The drawing under review shows one solid part. Ordinate dimensions are in mm from its lowest x, y, z. A direction names the side the tool comes from. Round coordinates to 2 decimals unless told otherwise and drop trailing zeros. Order: outer loops, then holes, each group sorted by start corner. A loop starts at its lowest first (then second) coordinate and runs counter-clockwise, first axis right, second up. Notation, with made-up numbers: M -33.5,60 L 0.5,60 A20 cw 0.5,93 Z; hole C -4.5,-16 d10. An arc over 180 degrees is marked long. Answer as a JSON object with one key per item and string values. Group by question number.
1. Add section A-A on z = 23.5. State the section outline as (x, y) points.
2. Add section D-D on z = 3. State the section outline as (x, y) points.
3. Add section C-C on y = 1. State the section outline as (x, z) points, and give its area (3 significant figures).
4. Clearance check with flat-ended pins moving along their axes: P1, Ø0.6, axis at x = 2.5, y = 1, coming from the -Z side; P2, Ø1, axis at x = 13, y = 3, coming from the -Z side (1 decimal); P3, Ø8, axis at x = 20.5, z = 33, coming from the +Y side; P4, Ø2, axis at x = 2.5, y = 1.5, coming from the +Z side. State where each tip first meets the part, or that it passes through.
5. To check wall thickness, follow probe 1 along X at (y, z) = (6.25, 24); probe 2 along Y at (x, z) = (34.5, 42.5); probe 3 along Z at (x, y) = (31, 7.25) (1 decimal). State the ranges of each line that lie inside material, in increasing order. Write a range as [from, to].
6. Mouldability with a two-part tool opening along X and no side actions: class the marked faces 3, 4 and 5 as released by +X, released by -X, zero draft, split by the parting line, or undercut.
7. Machinability: for the marked faces 1 and 2, which of the approach directions +Z, -Z, +X, -X, +Y, -Y give a long, thin tool a straight path to every point of the face, cutting with its end or side? Answer none if there is none.
8. Add section B-B on x = 16.5. State the section outline as (y, z) points (1 decimal).
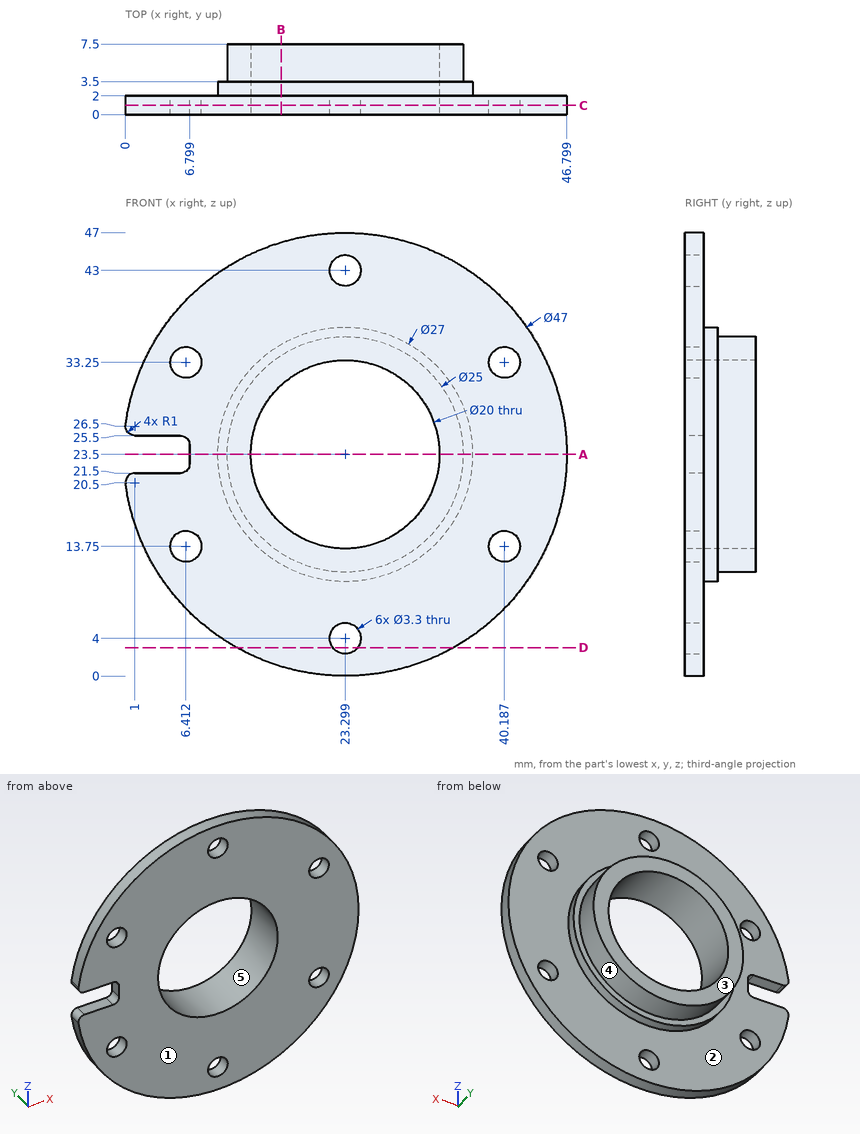
Recorded:
{
 "1": {"outline": "M 6.8,0 L 13.3,0 L 13.3,7.5 L 10.8,7.5 L 10.8,3.5 L 9.8,3.5 L 9.8,2 L 6.8,2 Z; M 33.3,0 L 46.8,0 L 46.8,2 L 36.8,2 L 36.8,3.5 L 35.8,3.5 L 35.8,7.5 L 33.3,7.5 Z"},
 "2": {"outline": "M 11.81,0 L 21.99,0 L 21.99,2 L 11.81,2 Z; M 24.61,0 L 34.79,0 L 34.79,2 L 24.61,2 Z"},
 "3": {"outline": "M 0.01,20.37 A23.5 ccw long 0.01,26.63 A1 ccw 1,25.5 L 5.8,25.5 A1 cw 6.8,24.5 L 6.8,22.5 A1 cw 5.8,21.5 L 1,21.5 A1 ccw Z; hole C 6.41,13.75 d3.3; hole C 6.41,33.25 d3.3; hole C 23.3,23.5 d20; hole C 23.3,4 d3.3; hole C 23.3,43 d3.3; hole C 40.19,13.75 d3.3; hole C 40.19,33.25 d3.3", "area": "1,340 mm²"},
 "4": {"P1": "stops at z = 12.01", "P2": "stops at z = 14.2", "P3": "stops at y = 7.5", "P4": "stops at z = 36.16"},
 "5": {"probe 1": "x = [10.81, 13.31], [33.29, 35.79]", "probe 2": "y = [0, 2]", "probe 3": "z = [13.7, 17.1], [29.9, 33.3]"},
 "6": {"face 3": "zero draft", "face 4": "split by the parting line", "face 5": "undercut"},
 "7": {"face 1": "+Z, -Z, +X, -X, -Y", "face 2": "+Y"},
 "8": {"outline": "M 0,1 L 2,1 L 2,11.8 L 3.5,11.8 L 3.5,13 L 7.5,13 L 7.5,16.2 L 0,16.2 Z; M 0,30.8 L 7.5,30.8 L 7.5,34 L 3.5,34 L 3.5,35.2 L 2,35.2 L 2,46 L 0,46 Z"}
}
